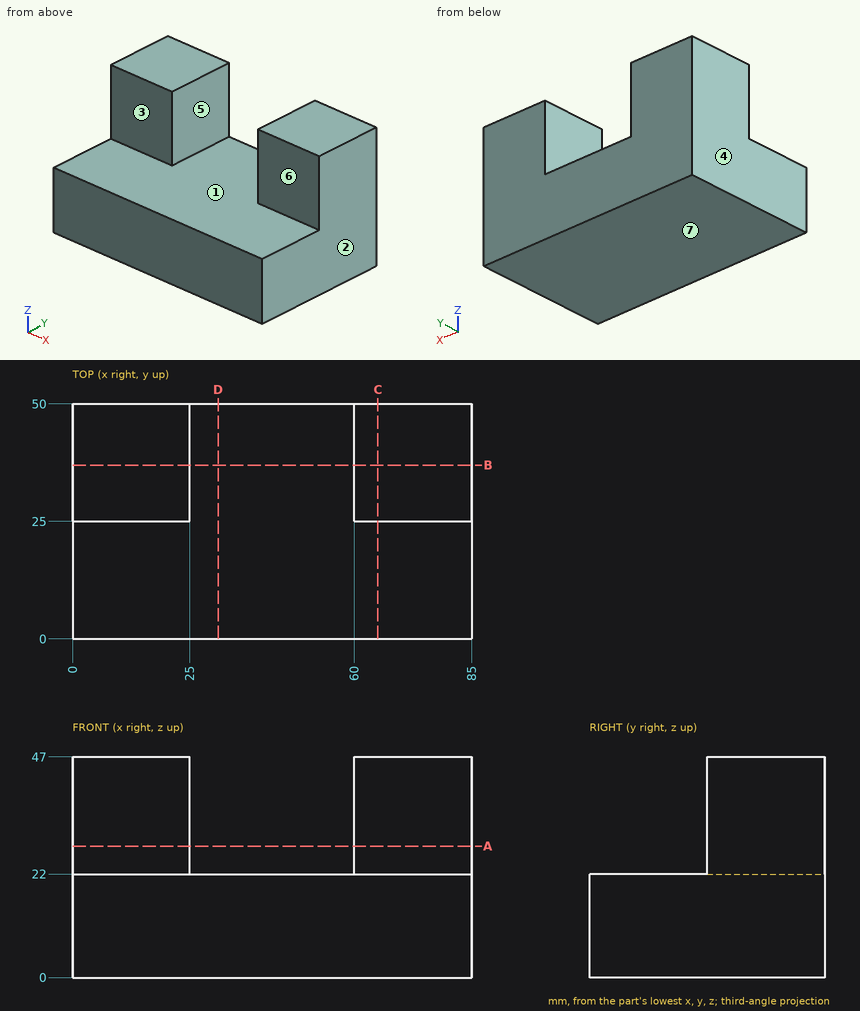
For this review, use the dimensioned drawing (mm, ordinates from the lowest corner) and the shaded views. A direction names the side the tool comes from. Give positions to 0.01 mm unless a question says otherwise; leave off trailing zeros. Loops run counter-clockwise (first coordinate to the right, second up) from the corner with the lowest first, then second, coordinate; pieces in that order, holes last. Notation, with made-up numbers: (50, -34.5) -> (64, -34.5) arc R34 ccw to (64, 1.5) -> close; hole circle Ø11 at (3.5, 37). An arc over 180 degrees is marked (long way). One line per question, with ' | ' between items. Start each with the question number.
(1) We need section A-A (z = 28). State the section outline as (x, y) points.
(2) For line 1 (X direction, y = 38.5, z = 31); line 2 (Z direction, x = 77, y = 21); line 3 (Y direction, x = 71.5, z = 35.5), list the stretches that pass through material, from the lowest coordinate up.
(3) For the marked faces 5, 6 and 7, list the 3-axis set-ups (+Z, -Z, +X, -X, +Y, -Y) from which the entire face can be reached by the end or side of a thin tool; tool diameter is ignored.
(4) Insertion check: P1, Ø1.5, axis at x = 31.5, y = 16, coming from the -Z side; P2, Ø6, axis at x = 43, y = 11.5, coming from the +Z side; P3, Ø7.5, axis at x = 18.5, z = 36, coming from the -Y side. Each pin has a flat end and moves straight along its axis. Give the tip position at first contact, or say it passes through.
(5) Draft analysis for pull direction X (two halves, no side actions). For the marked faces 1, 2, 3 and 4, state which applies: +X half, -X half, draft (parallel to the pull), parting line (faces both ways), or undercut.
(6) We need section B-B (y = 37). State the section outline as (x, z) points, and give its area (3 significant figures).
(7) We need section D-D (x = 31). State the section outline as (y, z) points, and give its area (3 significant figures).
(8) We need section C-C (x = 65). State the section outline as (y, z) points, and give its area (4 significant figures).
The answers:
1) outline: (0, 25) -> (25, 25) -> (25, 50) -> (0, 50) -> close; (60, 25) -> (85, 25) -> (85, 50) -> (60, 50) -> close
2) line 1: x = 0 to 25, 60 to 85 | line 2: z = 0 to 22 | line 3: y = 25 to 50
3) face 5: +Z, +Y, -Y | face 6: +Z, +X, -X, -Y | face 7: -Z, +X, -X, +Y, -Y
4) P1: stops at z = 0 | P2: stops at z = 22 | P3: stops at y = 25
5) face 1: undercut | face 2: +X half | face 3: draft | face 4: -X half
6) outline: (0, 0) -> (85, 0) -> (85, 47) -> (60, 47) -> (60, 22) -> (25, 22) -> (25, 47) -> (0, 47) -> close | area: 3,120 mm^2
7) outline: (0, 0) -> (50, 0) -> (50, 22) -> (0, 22) -> close | area: 1,100 mm^2
8) outline: (0, 0) -> (50, 0) -> (50, 47) -> (25, 47) -> (25, 22) -> (0, 22) -> close | area: 1,725 mm^2
